from build123d import *

# Parameters (mm, degrees)
SKETCH_1_W          = 65.6
SKETCH_1_H          = 123.6
EXTRUDE_1_DEPTH     = 2
CUT_EXTRUDE_3_DEPTH = 3.2
SKETCH_3_W          = 54
SKETCH_3_H          = 78
CUT_EXTRUDE_2_DEPTH = 1
FILLET_1_R          = 1


with BuildPart() as part:
    # 草图1 → 凸台-拉伸1 (new body)
    with BuildSketch(Plane(origin=(0, 0, 0), x_dir=(1, 0, 0), z_dir=(0, 1, 0))):
        with Locations((0, -64)):
            Rectangle(SKETCH_1_W, SKETCH_1_H)
    extrude(amount=-EXTRUDE_1_DEPTH)

    # 草图4 → 切除-拉伸3 (cut, symmetric)
    with BuildSketch(Plane(origin=(0, 0, 0), x_dir=(0, 0, -1), z_dir=(1, 0, 0))):
        Polygon((-125.8, 0), (-124.645299462, -2), (-125.8, -2), align=None)
        Polygon((-2.2, 0), (-2.2, -2), (-3.354700538, -2), align=None)
    extrude(amount=CUT_EXTRUDE_3_DEPTH, both=True, mode=Mode.SUBTRACT)

    # 草图3 → 切除-拉伸2 (cut)
    with BuildSketch(Plane(origin=(0, 0, 0), x_dir=(1, 0, 0), z_dir=(0, 1, 0))):
        with Locations((0, -80)):
            Rectangle(SKETCH_3_W, SKETCH_3_H)
    extrude(amount=-CUT_EXTRUDE_2_DEPTH, mode=Mode.SUBTRACT)

    # 圆角1
    fillet_1_edges = [part.edges().sort_by_distance(p)[0] for p in [
        (32.8, -1, 125.8),
        (32.8, -1, 2.2),
        (-32.8, -1, 2.2),
        (-32.8, -1, 125.8),
    ]]
    fillet(fillet_1_edges, radius=FILLET_1_R)


solid = part.part
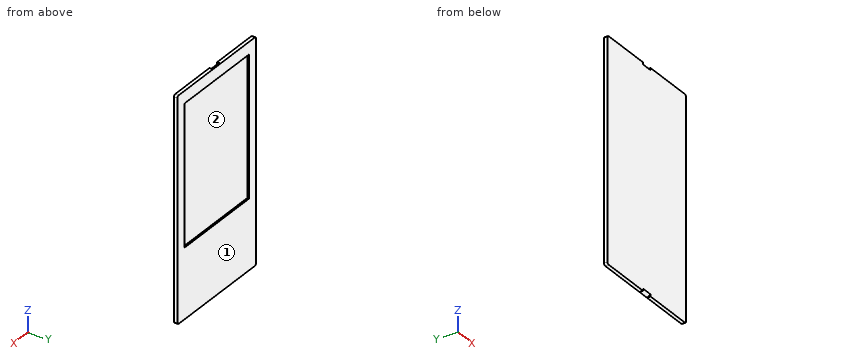
Geometry: final body of the model. Coordinates: model frame, mm. Face numbers are marked on the shaded views. Give positions to 0.01 mm unless a question says otherwise; leave off trailing zeros. Loops run counter-clockwise (first coordinate to the right, second up) from the corner with the lowest first, then second, coordinate; pieces in that order, holes last. Notation, with made-up numbers: M 30,63 L 70,63 A23 ccw 70,80 Z; hole C -37.75,72 d2. An arc over 180 degrees is marked long. Put each result on its own line as item: value.
1) Cut plane C-C, the plane z = 59.5. Return the cut outline in (x, y).
Computed values:
outline: M -32.8,-2 L 32.8,-2 L 32.8,0 L 27,0 L 27,-1 L -27,-1 L -27,0 L -32.8,0 Z
2) Cut plane A-A, the plane x = -1.5. Return the cut outline in (y, z), plus the area to 3 significant figures.
Computed values:
outline: M -2,3.35 L 0,2.2 L 0,41 L -1,41 L -1,119 L 0,119 L 0,125.8 L -2,124.65 Z
area: 167 mm^2
3) Material intervals for L1, parallel to X at y = -0.7, z = 94; L2, parallel to Z at x = 9, y = -0.1; L3, parallel to Y at x = 20.5, z = 68, sorted ascending. Write a range as from..to.
Computed values:
L1: x = -32.8..-27, 27..32.8
L2: z = 2.2..41, 119..125.8
L3: y = -2..-1
4) Cut plane B-B, the plane y = -0.4. Return the cut outline in (x, z).
Computed values:
outline: M -32.8,3.2 A1 ccw -31.8,2.2 L -3.2,2.2 L -3.2,2.43 L 3.2,2.43 L 3.2,2.2 L 31.8,2.2 A1 ccw 32.8,3.2 L 32.8,124.8 A1 ccw 31.8,125.8 L 3.2,125.8 L 3.2,125.57 L -3.2,125.57 L -3.2,125.8 L -31.8,125.8 A1 ccw -32.8,124.8 Z; hole M -27,41 L 27,41 L 27,119 L -27,119 Z
5) First-contact query: P1, Ø0.9, axis at y = -1, z = 125.5, coming from the +X side; P2, Ø6, axis at x = -23.5, z = 83.5, coming from the +Y side; P3, Ø0.5, axis at x = 2, y = -0.5, coming from the +Z side. Flat tips, straight axial feed; report the tip coordinate or a pass-through.
Computed values:
P1: stops at x = 32.77
P2: stops at y = -1
P3: stops at z = 125.66
6) Mould query, pull axis Z, two halves, no side actions, for the marked faces 1 and 2. Classes: released by +Z, released by -Z, zero draft, split by the parting line, or undercut.
Computed values:
face 1: zero draft
face 2: undercut
